from build123d import *

# Parameters (mm, degrees)
F0_W        = 39.3818542361
F0_H        = 94.9496030807
F1_DEPTH    = 25.4
F2_T1_DEPTH = 152.4
F3_T1_DEPTH = 101.2996030808
F3_T4_ANGLE = 148.6516311692
F3_T6_ANGLE = 148.6516311692


# Not quite as in the source:
# - a fillet or chamfer that OpenCascade refuses, or shapes differently, is made with other operations: its cross-section is extruded or revolved along the edge and cut away or added


with BuildPart() as f1:
    # F0 (on Top) → F1 (new body)
    with BuildSketch(Plane.XY):
        Rectangle(F0_W, F0_H)
    extrude(amount=F1_DEPTH)

    # F2: fillet of radius 25.4 on 2 edges, made by hand

    # F2_s2 → F2_t1 (cut)
    with BuildSketch(Plane.XY.offset(-63.5)):
        with BuildLine():
            ThreePointArc((-5.7090728819, -47.4748015404), (12.2514393602, -40.0353137825), (19.6909271181, -22.0748015404))
            Line((19.6909271181, -22.0748015404), (19.6909271181, -47.4748015404))
            Line((19.6909271181, -47.4748015404), (-5.7090728819, -47.4748015404))
        make_face()
        with BuildLine():
            ThreePointArc((5.7090728819, -47.4748015404), (-12.2514393602, -40.0353137825), (-19.6909271181, -22.0748015404))
            Line((-19.6909271181, -22.0748015404), (-19.6909271181, -47.4748015404))
            Line((-19.6909271181, -47.4748015404), (5.7090728819, -47.4748015404))
        make_face()
    extrude(amount=F2_T1_DEPTH, mode=Mode.SUBTRACT)

    # F3: fillet of radius 12.7 on 4 edges, made by hand

    # F3_s2 → F3_t1 (cut)
    with BuildSketch(Plane.XZ.offset(-79.2248015404)):
        with BuildLine():
            ThreePointArc((6.9909271181, 25.4), (15.9711832391, 21.6802561211), (19.6909271181, 12.7))
            Line((19.6909271181, 12.7), (19.6909271181, 25.4))
            Line((19.6909271181, 25.4), (6.9909271181, 25.4))
        make_face()
        with BuildLine():
            ThreePointArc((-19.6909271181, 12.7), (-15.9711832391, 21.6802561211), (-6.9909271181, 25.4))
            Line((-6.9909271181, 25.4), (-19.6909271181, 25.4))
            Line((-19.6909271181, 25.4), (-19.6909271181, 12.7))
        make_face()
    extrude(amount=F3_T1_DEPTH, mode=Mode.SUBTRACT)

    # F3_s3 → F3_t4 (revolve, cut)
    with BuildSketch(Plane.XZ.offset(22.0748015403)):
        with BuildLine():
            ThreePointArc((6.9909271181, 25.4), (15.9711832392, 21.6802561211), (19.6909271181, 12.7))
            Line((19.6909271181, 12.7), (19.6909271181, 25.4))
            Line((19.6909271181, 25.4), (6.9909271181, 25.4))
        make_face()
    revolve(axis=Axis((-5.709072882, -22.0748015403, 25.4), (0, 0, -1)), revolution_arc=F3_T4_ANGLE, mode=Mode.SUBTRACT)

    # F3_s5 → F3_t6 (revolve, cut)
    with BuildSketch(Plane(origin=(-8.2625761257, -13.5637424397, 0), x_dir=(0, 0, 1), z_dir=(0.5202402568, 0.8540199501, 0))):
        with BuildLine():
            ThreePointArc((12.7, 41.759862561), (21.6802561211, 38.040118682), (25.4, 29.059862561))
            Line((25.4, 29.059862561), (25.4, 41.759862561))
            Line((25.4, 41.759862561), (12.7, 41.759862561))
        make_face()
    revolve(axis=Axis((5.709072882, -22.0748015403, 25.4), (0, 0, -1)), revolution_arc=F3_T6_ANGLE, mode=Mode.SUBTRACT)


solid = f1.part
Verification items for the finished model (mm, model axes). Coordinates: 2 decimals unless noted, no trailing zeros. Order: outer loops, then holes, each group sorted by start corner. A loop starts at its lowest first (then second) coordinate and runs counter-clockwise, first axis right, second up. Notation, with made-up numbers: M -19.75,42.25 L 17.25,42.25 A24 cw 17.25,59.25 Z; hole C -15,81 d8. An arc over 180 degrees is marked long. Return JSON: item names as keys, results as strings.
1) Cross-section at B-B, the plane y = 12.5. Record the boundary of the cut face in (x, z), and give its area (3 significant figures).
Answer list:
{"outline": "M -19.69,0 L 19.69,0 L 19.69,12.7 A12.7 ccw 6.99,25.4 L -6.99,25.4 A12.7 ccw -19.69,12.7 Z", "area": "931 mm2"}
2) Gauge pin test, flat ends, axial feed: pin 1 (8 mm diameter, centred on x = -11, z = 13, fed in from -Y); pin 2 (1 mm diameter, centred on x = -2.5, z = 21, fed in from -Y); pin 3 (5 mm diameter, centred on y = -20.5, z = 19, fed in from -X). Record the tip position at first contact, or that the pin passes through.
Answer list:
{"pin 1": "y = -44.06", "pin 2": "y = -43.3", "pin 3": "x = -19.11"}
3) Cross-section at A-A, the plane z = 5.25. Record the boundary of the cut face in (x, y).
Answer list:
{"outline": "M -19.69,-22.07 A25.4 ccw 0,-46.82 A25.4 ccw 19.69,-22.07 L 19.69,47.47 L -19.69,47.47 Z"}
4) Thickness scan on L1, parallel to Z at x = 7.5, y = 5; L2, parallel to X at y = 22, z = 18.25; L3, parallel to Y at x = -9, z = 4.5. Record the ranges inside material, lowest first. Write a range as [from, to].
Answer list:
{"L1": "[0, 25.39]", "L2": "[-18.41, 18.41]", "L3": "[-42.78, 47.47]"}
5) Cross-section at C-C, the plane z = 17.75. Record the boundary of the cut face in (x, y).
Answer list:
{"outline": "M -18.64,-22.07 A24.35 ccw 0,-45.75 A24.35 ccw 18.64,-22.07 L 18.64,47.47 L -18.64,47.47 Z"}
